Build history of the part. All positions in model axes, mm. Coordinates: 2 decimals unless noted, no trailing zeros. Write each loop counter-clockwise with the first axis right and the second up, starting at its lowest first coordinate (ties: lowest second). Pieces come first, ordered by that corner, then holes. Notation, with made-up numbers: M 20,75.5 L 27,75.5 A4 ccw 27,81.5 Z; hole C 89,80 d8. An arc over 180 degrees is marked long. Use CSV: the item, a comma, the result in double quotes. Start each with the question number.
```python
from build123d import *

# Parameters (mm, degrees)
SKETCH1_W           = 139
SKETCH1_H           = 160
BOSS_EXTRUDE1_DEPTH = 5
SKETCH2_W           = 16
SKETCH2_H           = 16
CUT_EXTRUDE1_DEPTH  = 5
SKETCH3_R           = 2.15
CUT_EXTRUDE2_DEPTH  = 5
SKETCH4_R           = 2.15
CUT_EXTRUDE3_DEPTH  = 5
LPATTERN1_COUNT     = 4
LPATTERN1_PITCH     = 35
SKETCH5_R           = 2.15
CUT_EXTRUDE4_DEPTH  = 5
SKETCH6_W           = 109
SKETCH6_H           = 15
BOSS_EXTRUDE2_DEPTH = 5
SKETCH7_W           = 55
SKETCH7_H           = 104
CUT_EXTRUDE5_DEPTH  = 5
SKETCH8_R           = 2.15
CUT_EXTRUDE6_DEPTH  = 5
FILLET1_R           = 3


with BuildPart() as part:
    # Sketch1 → Boss-Extrude1 (new body)
    with BuildSketch(Plane.XY):
        with Locations((69.5, 80)):
            Rectangle(SKETCH1_W, SKETCH1_H)
    extrude(amount=BOSS_EXTRUDE1_DEPTH)

    # Sketch2 → Cut-Extrude1 (cut)
    with BuildSketch(Plane.XY.offset(5)):
        with Locations((131, 152)):
            Rectangle(SKETCH2_W, SKETCH2_H)
        with Locations((8, 152)):
            Rectangle(SKETCH2_W, SKETCH2_H)
    extrude(amount=-CUT_EXTRUDE1_DEPTH, mode=Mode.SUBTRACT)

    # Sketch3 → Cut-Extrude2 (cut)
    with BuildSketch(Plane.XY.offset(5)):
        with Locations((69.5, 152.5)):
            Circle(SKETCH3_R)
        with Locations((44.5, 152.5)):
            Circle(SKETCH3_R)
        with Locations(Location((94.5, 152.5, 0), (0, 0, 180))):
            Circle(SKETCH3_R)
    extrude(amount=-CUT_EXTRUDE2_DEPTH, mode=Mode.SUBTRACT)

    # Sketch4 → Cut-Extrude3 (cut)
    with BuildSketch(Plane.XY.offset(5)):
        with Locations((131.5, 129)):
            Circle(SKETCH4_R)
        with Locations(Location((7.5, 129, 0), (0, 0, 180))):
            Circle(SKETCH4_R)
    cut_extrude3 = extrude(amount=-CUT_EXTRUDE3_DEPTH, mode=Mode.SUBTRACT)

    # LPattern1: Cut-Extrude3 ×4
    with Locations(*[(0, -i * LPATTERN1_PITCH, 0) for i in range(1, LPATTERN1_COUNT)]):
        add(cut_extrude3, mode=Mode.SUBTRACT)

    # Sketch5 → Cut-Extrude4 (cut)
    with BuildSketch(Plane.XY.offset(5)):
        with Locations((117, 112)):
            Circle(SKETCH5_R)
        with Locations((117, 87)):
            Circle(SKETCH5_R)
        with Locations(Location((22, 87, 0), (0, 0, 180))):
            Circle(SKETCH5_R)
        with Locations(Location((22, 112, 0), (0, 0, 180))):
            Circle(SKETCH5_R)
    extrude(amount=-CUT_EXTRUDE4_DEPTH, mode=Mode.SUBTRACT)

    # Sketch6 → Boss-Extrude2 (add)
    with BuildSketch(Plane(origin=(0, 0, 0), x_dir=(-1, 0, 0), z_dir=(0, 0, -1))):
        with Locations((-69.5, -7.5)):
            Rectangle(SKETCH6_W, SKETCH6_H)
    extrude(amount=-BOSS_EXTRUDE2_DEPTH)

    # Sketch7 → Cut-Extrude5 (cut)
    with BuildSketch(Plane.XY.offset(5)):
        with Locations((69.5, 47)):
            Rectangle(SKETCH7_W, SKETCH7_H)
    extrude(amount=-CUT_EXTRUDE5_DEPTH, mode=Mode.SUBTRACT)

    # Sketch8 → Cut-Extrude6 (cut)
    with BuildSketch(Plane.XY.offset(5)):
        with Locations((102, 5)):
            Circle(SKETCH8_R)
        with Locations((102, 120)):
            Circle(SKETCH8_R)
        with Locations(Location((37, 120, 0), (0, 0, 180))):
            Circle(SKETCH8_R)
        with Locations(Location((37, 5, 0), (0, 0, 180))):
            Circle(SKETCH8_R)
    extrude(amount=-CUT_EXTRUDE6_DEPTH, mode=Mode.SUBTRACT)

    # Fillet1
    fillet1_edges = [part.edges().sort_by_distance(p)[0] for p in [
        (124, -15, 2.5),
        (15, -15, 2.5),
        (139, 144, 2.5),
        (123, 160, 2.5),
        (16, 160, 2.5),
        (0, 144, 2.5),
        (139, 0, 2.5),
        (0, 0, 2.5),
    ]]
    fillet(fillet1_edges, radius=FILLET1_R)


solid = part.part
```
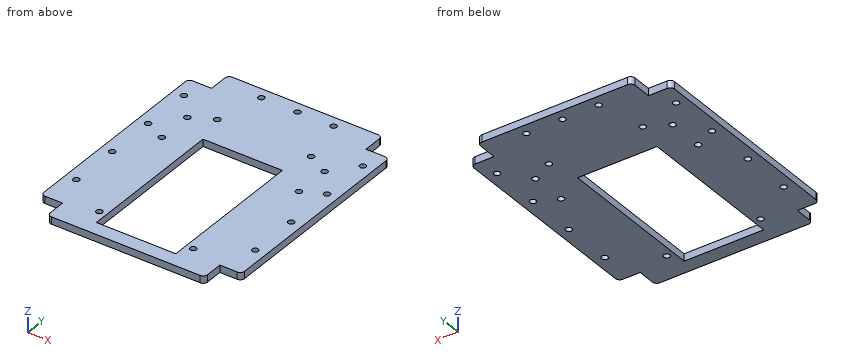
1. Slice it at B-B (x = 131.5). List the corners of the cut face in (y, z), and give its area (3 significant figures).
2. Slice it at C-C (y = 5). List the corners of the cut face in (x, z), and give its area (3 significant figures).
3. Slice it at A-A (x = 102). List the corners of the cut face in (y, z).
4. Drill centre lines: line 1 along X through (y, z) = (24, 1.3); line 2 along X through (y, z) = (152.5, 2.8); line 3 along Y through (x, z) = (7.5, 1.5). Where is each one in solid material? Low to high. Write a range as from..to.
5. Slice it at D-D (y = 54). List the corners of the cut face in (x, z), and give its area (3 significant figures).
6. Flat gauge pins, fed straight in: pin 1 (4 mm diameter, centred on x = 7.5, y = 94, fed in from +Z); pin 2 (5.5 mm diameter, centred on x = 131.5, y = 59, fed in from -Z); pin 3 (2.5 mm diameter, centred on y = 149, z = 3.5, fed in from -X). Where does each tip first touch, or does it go through?
Established:
1,outline,"M 0,0 L 21.85,0 L 21.85,5 L 0,5 Z; M 26.15,0 L 56.85,0 L 56.85,5 L 26.15,5 Z; M 61.15,0 L 91.85,0 L 91.85,5 L 61.15,5 Z; M 96.15,0 L 126.85,0 L 126.85,5 L 96.15,5 Z; M 131.15,0 L 144,0 L 144,5 L 131.15,5 Z"
1,area,"634 mm2"
2,outline,"M 0,0 L 34.85,0 L 34.85,5 L 0,5 Z; M 39.15,0 L 42,0 L 42,5 L 39.15,5 Z; M 97,0 L 99.85,0 L 99.85,5 L 97,5 Z; M 104.15,0 L 139,0 L 139,5 L 104.15,5 Z"
2,area,"377 mm2"
3,outline,"M -15,0 L 2.85,0 L 2.85,5 L -15,5 Z; M 7.15,0 L 117.85,0 L 117.85,5 L 7.15,5 Z; M 122.15,0 L 160,0 L 160,5 L 122.15,5 Z"
4,line 1,"x = 0..5.35, 9.65..42, 97..129.35, 133.65..139"
4,line 2,"x = 16..42.35, 46.65..67.35, 71.65..92.35, 96.65..123"
4,line 3,"y = 0..21.85, 26.15..56.85, 61.15..91.85, 96.15..126.85, 131.15..144"
5,outline,"M 0,0 L 42,0 L 42,5 L 0,5 Z; M 97,0 L 139,0 L 139,5 L 97,5 Z"
5,area,"420 mm2"
6,pin 1,"passes through"
6,pin 2,"stops at z = 0"
6,pin 3,"stops at x = 16"
